Geometry: final body of the model. Coordinates: model frame, mm. Face numbers are marked on the shaded views. A direction names the side the tool comes from. Round coordinates to 2 decimals unless told otherwise and drop trailing zeros. Loops run counter-clockwise (first coordinate to the right, second up) from the corner with the lowest first, then second, coordinate; pieces in that order, holes last. Notation, with made-up numbers: (-31.5, 15) -> (25.5, 15) arc R25 ccw to (25.5, 27) -> close; hole circle Ø11 at (-24, -8). An arc over 180 degrees is marked (long way). Answer in a Markdown table with one row per item.
```python
from build123d import *

# Parameters (mm, degrees)
SKICA1_R                 = 50
VYSUNOUT1_DEPTH          = 5
SKICA3_R                 = 5
ODEBRAT_VYSUNUT_M1_DEPTH = 6
KRUHOV_POLE1_COUNT       = 9
VYSUNOUT2_DEPTH          = 10
ZAOBLIT2_R               = 10
ODEBRAT_VYSUNUT_M2_REACH = 17
SKICA5_R                 = 4


with BuildPart() as part:
    # Skica1 → Vysunout1 (new body)
    with BuildSketch(Plane.XY):
        Circle(SKICA1_R)
    extrude(amount=VYSUNOUT1_DEPTH)

    # Skica3 → Odebrat vysunutím1 (cut, through all)
    with BuildSketch(Plane.XY.offset(5)):
        with Locations((-40, 0)):
            Circle(SKICA3_R)
    odebrat_vysunut_m1 = extrude(amount=-ODEBRAT_VYSUNUT_M1_DEPTH, mode=Mode.SUBTRACT)

    # Kruhové pole1: Odebrat vysunutím1 ×9 about axis
    kruhov_pole1_axis = Axis((0, 0, 0), (0, 0, 1))
    for i in range(1, KRUHOV_POLE1_COUNT):
        add(odebrat_vysunut_m1.rotate(kruhov_pole1_axis, i * 360 / KRUHOV_POLE1_COUNT), mode=Mode.SUBTRACT)

    # Skica2 → Vysunout2 (add)
    with BuildSketch(Plane.XY.offset(5)):
        Polygon((0, 28.284271247), (-28.284271247, 0), (0, -28.284271247), (28.284271247, 0), align=None)
    extrude(amount=VYSUNOUT2_DEPTH)

    # Zaoblit2
    zaoblit2_edges = [part.edges().sort_by_distance(p)[0] for p in [
        (-28.284271247, 0, 10),
        (0, -28.284271247, 10),
        (28.284271247, 0, 10),
        (0, 28.284271247, 10),
    ]]
    fillet(zaoblit2_edges, radius=ZAOBLIT2_R)

    # Skica5 → Odebrat vysunutím2 (cut, up to next)
    with BuildSketch(Plane.XY.offset(15), mode=Mode.PRIVATE) as odebrat_vysunut_m2_sk1:
        with Locations((19.460353897, 0)):
            Circle(SKICA5_R)
    odebrat_vysunut_m2_tool1 = extrude(odebrat_vysunut_m2_sk1.sketch, amount=-ODEBRAT_VYSUNUT_M2_REACH, mode=Mode.PRIVATE) & part.part
    add(odebrat_vysunut_m2_tool1.solids().sort_by_distance((19.460354, 0, 15))[0], mode=Mode.SUBTRACT)


solid = part.part
```
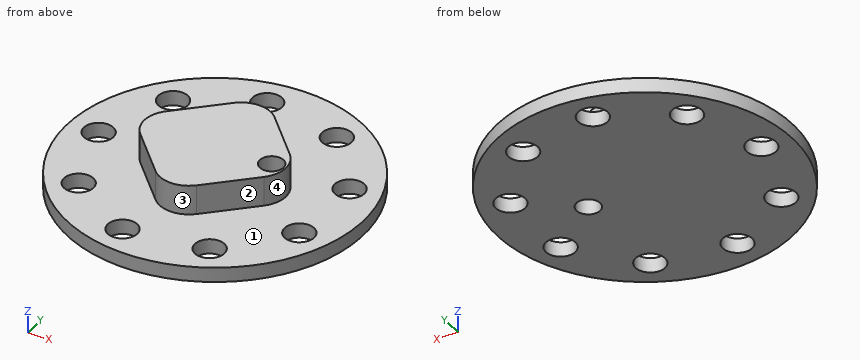
Item 1: Pin query (flat end, axial travel): pin 1 Ø6.5 at (x, y) = (19.46, 0) entering from -Z; pin 2 Ø8 at (x, z) = (14.5, 9.5) entering from +Y; pin 3 Ø3 at (x, y) = (26.5, 4) entering from +Z; pin 4 Ø2 at (y, z) = (8, 3) entering from +X. Return the tip coordinate at first contact, or that it passes through.
Answer:
| item | result |
|---|---|
| pin 1 | passes through |
| pin 2 | stops at y = 17.78 |
| pin 3 | stops at z = 5 |
| pin 4 | stops at x = 49.51 |
Item 2: Cut plane B-B (y = 0). Output: boundary loops of the cut face in (x, z), then the cut area to 3 significant figures.
Answer:
| item | result |
|---|---|
| outline | (-50, 0) -> (-45, 0) -> (-45, 5) -> (-50, 5) -> close; (-35, 0) -> (15.46, 0) -> (15.46, 15) -> (-24.14, 15) -> (-24.14, 5) -> (-35, 5) -> close; (23.46, 0) -> (50, 0) -> (50, 5) -> (24.14, 5) -> (24.14, 15) -> (23.46, 15) -> close |
| area | 813 mm² |
Item 3: Cut plane D-D (y = 26). Output: boundary loops of the cut face in (x, z), then the cut area to 3 significant figures.
Answer:
| item | result |
|---|---|
| outline | (-42.71, 0) -> (-35.63, 0) -> (-35.63, 5) -> (-42.71, 5) -> close; (-25.65, 0) -> (42.71, 0) -> (42.71, 5) -> (-25.65, 5) -> close |
| area | 377 mm² |
Item 4: Cut plane C-C (z = 6.5). Output: boundary loops of the cut face in (x, y), then the cut area to 3 significant figures.
Answer:
| item | result |
|---|---|
| outline | (-21.21, -7.07) -> (-7.07, -21.21) arc R10 ccw to (7.07, -21.21) -> (21.21, -7.07) arc R10 ccw to (21.21, 7.07) -> (7.07, 21.21) arc R10 ccw to (-7.07, 21.21) -> (-21.21, 7.07) arc R10 ccw to start; hole circle Ø8 at (19.46, 0) |
| area | 1,460 mm² |
Item 5: Line query: probe 1 along X at (y, z) = (-38.5, 1.25); probe 2 along Z at (x, y) = (-34, -5); probe 3 along X at (y, z) = (-33, 4.5). Output: solid intervals per line, ascending. Write a range as [from, to].
Answer:
| item | result |
|---|---|
| probe 1 | x = [-31.9, -11.87], [-2.03, 16.82], [23.18, 31.9] |
| probe 2 | z = [0, 5] |
| probe 3 | x = [-37.56, 15.28], [24.72, 37.56] |
Item 6: Cut plane A-A (x = -40). Output: boundary loops of the cut face in (y, z).
Answer:
| item | result |
|---|---|
| outline | (-30, 0) -> (-5, 0) -> (-5, 5) -> (-30, 5) -> close; (5, 0) -> (30, 0) -> (30, 5) -> (5, 5) -> close |
Item 7: Reachability of the marked faces 1, 2, 3 and 4 from +Z, -Z, +X, -X, +Y, -Y: full face, straight path, thin tool, end or side. Return the list, or none.
Answer:
| item | result |
|---|---|
| face 1 | +Z |
| face 2 | +Z, +X, -Y |
| face 3 | +Z, -Y |
| face 4 | +Z, +X |
